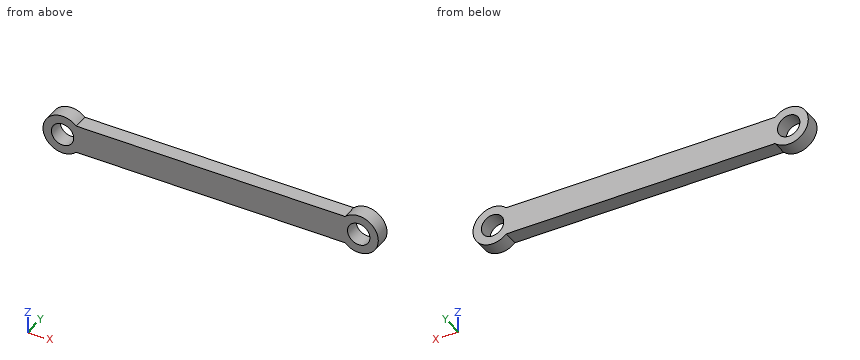
Autodesk Inventor part; units mm, degrees
ref_plane "YZ Plane" through (0, 0, 0) normal (1, 0, 0) x (0, 1, 0)
ref_plane "XZ Plane" through (0, 0, 0) normal (0, 1, 0) x (-1, 0, 0)
ref_plane "XY Plane" through (0, 0, 0) normal (0, 0, 1) x (1, 0, 0)
sketch "Sketch1" plane through (0, 0, 0) normal (0, 1, 0) x (-1, 0, 0)
  line L0 (0, 0) -> (57, 0)
  line L1 (57, 0) -> (57, 5)
  line L2 (57, 5) -> (0, 5)
  line L3 (0, 5) -> (0, 0)
  circle A0 centre (55, 2.5) radius 2
  circle A1 centre (2, 2.5) radius 2
  circle A2 centre (55, 2.5) radius 3.5
  circle A3 centre (2, 2.5) radius 3.5
  line L4 (57, 0) -> (57, 5)
  line L5 (57, 2.5) -> (0, 2.5)
  point P0 (52.5505, 0)
  point P1 (52.5505, 5)
  point P2 (4.4495, 5)
  point P3 (4.4495, 0)
  dimension "d0" = 5
  dimension "d1" = 57
  dimension "d2" = 4
  dimension "d3" = 4
  dimension "d4" = 7
  dimension "d5" = 7
extrude "Extrusion1" add sketch "Sketch1" along normal blind 2.7 contours L3 A1 L5 A3 L0 | L0 A3 L2 L3 | A3 L5 A2 L0 | L3 L2 A3 L5 A1 | A2 L5 A0 L1 L0 | L0 L1 L2 A2 | L2 A2 L5 A3 | A2 L2 L1 A0 L5
properties part number "FP V2 Batang Penggerak" material "Aluminum 6061"
The listing builds one solid part. Answer for the finished solid, in the listing's coordinates (mm). Round coordinates to 2 decimals unless told otherwise and drop trailing zeros. Write each loop counter-clockwise with the first axis right and the second up, starting at its lowest first coordinate (ties: lowest second). Pieces come first, ordered by that corner, then holes. Notation, with made-up numbers: (14, -23) - (59, -23) arc R31 ccw to (59, 16) - close; hole circle Ø9 at (31, -23.75). An arc over 180 degrees is marked (long way). Use a Markdown table: item, result. Add a question column.
1. Consider line 1 (X direction, y = 2.25, z = 2.5); line 2 (Z direction, x = -55, y = 1.2); line 3 (X direction, y = 0.2, z = 1.5). Determine where each line is inside the solid, lowest interval first.
2. The part is cut by section C-C (y = 0.7). Write down the section's boundary in (x, z).
3. The part is cut by section B-B (z = 2.5). Write down the section's boundary in (x, y), and give its area (3 significant figures).
4. The part is cut by section A-A (x = -55). Write down the section's boundary in (y, z).
5. The part is cut by section D-D (x = -7). Write down the section's boundary in (y, z), and give its area (3 significant figures).
6. Flat-ended cylindrical pins translate along their axes: P1, Ø0.8, axis at x = -26.5, y = 2, coming from the +Z side; P2, Ø1.4, axis at x = -34.5, y = 2, coming from the -Z side. Find the tip coordinate at first contact, or state that the pin passes through.
Reported:
| question | item | result |
|---|---|---|
| 1 | line 1 | -58.5 to -57, -53 to -4, 0 to 1.5 |
| 1 | line 2 | -1 to 0.5, 4.5 to 6 |
| 1 | line 3 | -58.35 to -56.73, -53.27 to -3.73, -0.27 to 1.35 |
| 2 | outline | (-52.55, 0) - (-4.45, 0) arc R3.5 ccw (long way) to (-4.45, 5) - (-52.55, 5) arc R3.5 ccw (long way) to start; hole circle Ø4 at (-55, 2.5); hole circle Ø4 at (-2, 2.5) |
| 3 | outline | (-58.5, 0) - (-57, 0) - (-57, 2.7) - (-58.5, 2.7) - close; (-53, 0) - (-4, 0) - (-4, 2.7) - (-53, 2.7) - close; (0, 0) - (1.5, 0) - (1.5, 2.7) - (0, 2.7) - close |
| 3 | area | 140 mm^2 |
| 4 | outline | (0, -1) - (2.7, -1) - (2.7, 0.5) - (0, 0.5) - close; (0, 4.5) - (2.7, 4.5) - (2.7, 6) - (0, 6) - close |
| 5 | outline | (0, 0) - (2.7, 0) - (2.7, 5) - (0, 5) - close |
| 5 | area | 13.5 mm^2 |
| 6 | P1 | z = 5 |
| 6 | P2 | z = 0 |
